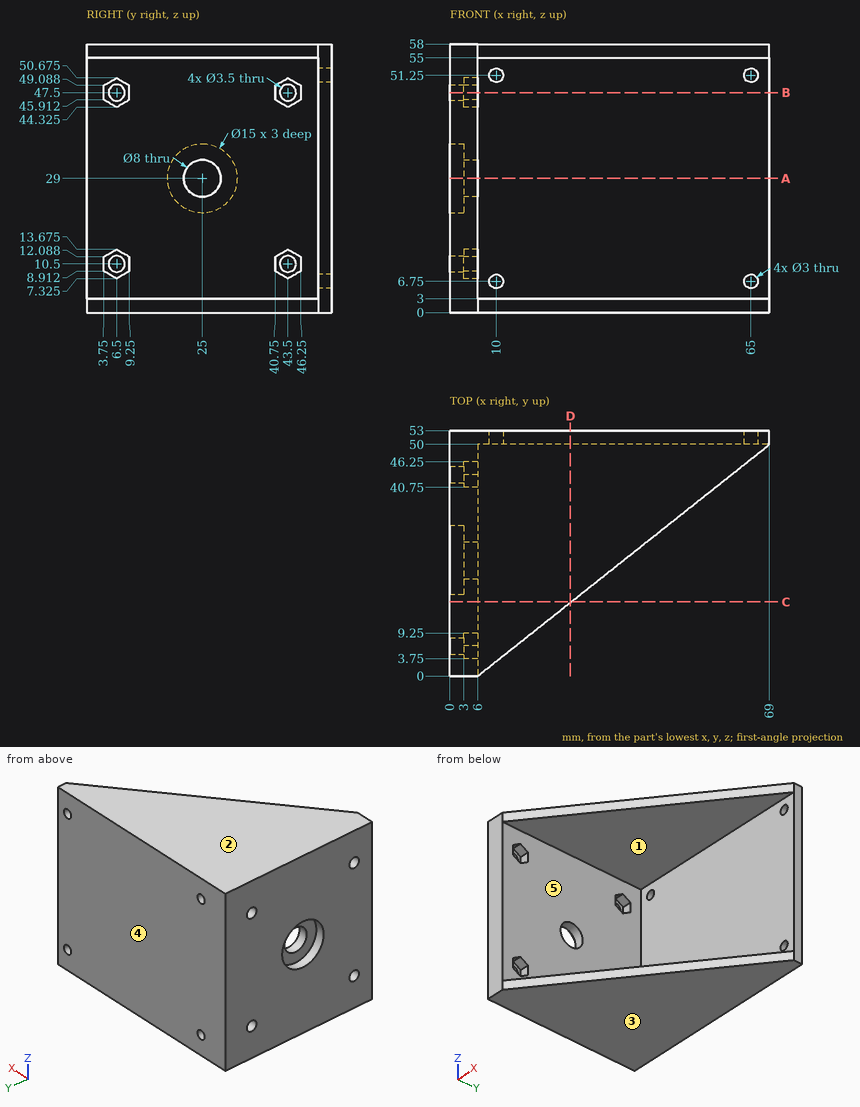
Can you work these out from the drawing? Everything is in mm from the part's minimum corner. A direction names the side the tool comes from. Give positions to 0.01 mm unless a question says otherwise; leave off trailing zeros. Loops run counter-clockwise (first coordinate to the right, second up) from the corner with the lowest first, then second, coordinate; pieces in that order, holes last. Notation, with made-up numbers: (-17.5, -31) -> (-13.5, -31) arc R28 cw to (-13.5, -12) -> close; hole circle Ø4 at (0.25, -29.5). An arc over 180 degrees is marked (long way). Write item = value, one per line.
1) Will these pins go through, and if not, where does the flat tip stop? pin 1 (12 mm diameter, centred on x = 51.5, y = 40.5, fed in from -Z); pin 2 (5 mm diameter, centred on y = 7.5, z = 16.5, fed in from +X); pin 3 (1.6 mm diameter, centred on y = 42.5, z = 10.5, fed in from +X).
Check result:
pin_1 = 0
pin_2 = 6
pin_3 = 3
2) Suppose I cut it at C-C on y = 16. Write out the boundary of the cut face in (x, z), then the cut area to 3 significant figures.
Check result:
outline = (0, 0) -> (26.16, 0) -> (26.16, 3) -> (6, 3) -> (6, 55) -> (26.16, 55) -> (26.16, 58) -> (0, 58) -> close
area = 469 mm2
3) Thinking about a two-plate mould opening in Z: for the marked faces 1, 2 and 3, which applies, released by +Z, released by -Z, zero draft, split by the parting line, or undercut?
Check result:
face_1 = undercut
face_2 = released by +Z
face_3 = released by -Z
4) Suppose I cut it at B-B on z = 47.5. Write out the boundary of the cut face in (x, y).
Check result:
outline = (0, 0) -> (6, 0) -> (6, 3.75) -> (3, 3.75) -> (3, 4.75) -> (0, 4.75) -> close; (0, 8.25) -> (3, 8.25) -> (3, 9.25) -> (6, 9.25) -> (6, 40.75) -> (3, 40.75) -> (3, 41.75) -> (0, 41.75) -> close; (0, 45.25) -> (3, 45.25) -> (3, 46.25) -> (6, 46.25) -> (6, 50) -> (69, 50) -> (69, 53) -> (0, 53) -> close
5) For the marked faces 4 and 5, which set-ups out of +Z, -Z, +X, -X, +Y, -Y let a thin tool reach every point of the face, with its end or its side?
Check result:
face_4 = +Z, -Z, +X, -X, +Y
face_5 = +X, -Y
6) Suppose I cut it at A-A on z = 29. Write out the boundary of the cut face in (x, y).
Check result:
outline = (0, 0) -> (6, 0) -> (6, 21) -> (3, 21) -> (3, 17.5) -> (0, 17.5) -> close; (0, 32.5) -> (3, 32.5) -> (3, 29) -> (6, 29) -> (6, 50) -> (69, 50) -> (69, 53) -> (0, 53) -> close
7) Suppose I cut it at D-D on x = 26. Write out the boundary of the cut face in (y, z), then the cut area to 3 significant figures.
Check result:
outline = (15.87, 0) -> (53, 0) -> (53, 58) -> (15.87, 58) -> (15.87, 55) -> (50, 55) -> (50, 3) -> (15.87, 3) -> close
area = 379 mm2
8) I need wall thicknesses on L1, parallel to Z at x = 10, y = 51.7; L2, parallel to Z at x = 2, y = 43; L3, parallel to Z at x = 35, y = 32.5. Which ranges of each line are inside material? Lowest first, please. Write a range as from..to.
Check result:
L1 = 0..5.25, 8.25..49.75, 52.75..58
L2 = 0..8.82, 12.18..45.82, 49.18..58
L3 = 0..3, 55..58
